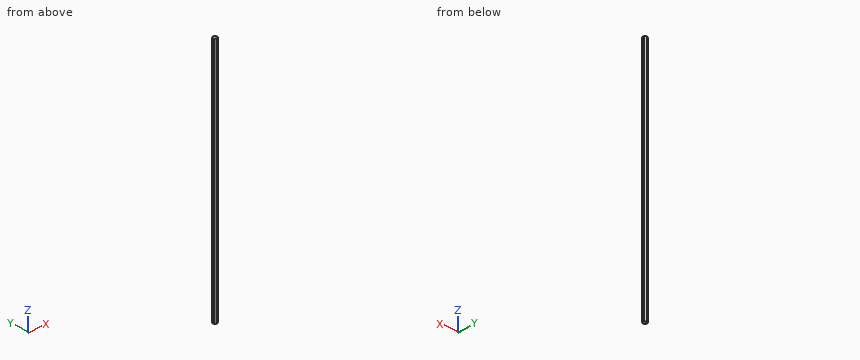
Autodesk Inventor part; units mm, degrees
ref_plane "YZ Plane" through (0, 0, 0) normal (1, 0, 0) x (0, 1, 0)
ref_plane "XZ Plane" through (0, 0, 0) normal (0, 1, 0) x (-1, 0, 0)
ref_plane "XY Plane" through (0, 0, 0) normal (0, 0, 1) x (1, 0, 0)
sketch "Sketch1" plane through (-2.1, -1.2124, 67.5) normal (0, 0, 1) x (1, 0, 0)
  line L0 (2.1, 4.0992) -> (4.6, 2.6558)
  line L1 (2.1, 3.6373) -> (0, 2.4249)
  line L2 (-0.4, 2.6558) -> (2.1, 4.0992)
  line L3 (-0.4, -0.2309) -> (-0.4, 2.6558)
  line L4 (2.1, -1.6743) -> (-0.4, -0.2309)
  line L5 (4.6, -0.2309) -> (2.1, -1.6743)
  line L6 (4.6, 2.6558) -> (4.6, -0.2309)
  point P0 (2.1, 1.2124)
extrude "Extrusion1" add sketch "Sketch1" against normal blind 317.5
sketch "Sketch2" plane through (-2.1, -1.2124, -250) normal (0, 0, -1) x (1, 0, 0)
  point P0 (2.1, -1.2124)
  point P1 (2.1, -1.2124)
properties part number "5mm axel"
Geometry: final body of the model. Coordinates: model frame, mm. Round coordinates to 2 decimals unless told otherwise and drop trailing zeros. Write each loop counter-clockwise with the first axis right and the second up, starting at its lowest first coordinate (ties: lowest second). Pieces come first, ordered by that corner, then holes. Notation, with made-up numbers: M 54.5,42.25 L 72.5,42.25 A31 cw 72.5,69.25 Z; hole C -32,-8.5 d3. An arc over 180 degrees is marked long. Write item = value, one per line.
Item 1: Material intervals for line 1 along Y through (x, z) = (-0.6, -142.5); line 2 along X through (y, z) = (1.8, -88.5); line 3 along X through (y, z) = (1.75, -161.5), sorted ascending. Write a range as [from, to].
Findings:
line_1 = [-2.54, 2.54]
line_2 = [-1.88, 1.88]
line_3 = [-1.97, 1.97]
Item 2: Section query A-A on z = 27.5. Return loops of the section in (x, y), then the cut area to 3 significant figures.
Findings:
outline = M -2.5,-1.44 L 0,-2.89 L 2.5,-1.44 L 2.5,1.44 L 0,2.89 L -2.5,1.44 Z
area = 21.7 mm^2
Item 3: Section query B-B on x = -1.7. Return loops of the section in (y, z), then the cut area to 3 significant figures.
Findings:
outline = M -1.91,-250 L 1.91,-250 L 1.91,67.5 L -1.91,67.5 Z
area = 1,210 mm^2
Item 4: Pin query (flat end, axial travel): P1, Ø1, axis at x = 1, z = -140, coming from the +Y side. Return the tip coordinate at first contact, or that it passes through.
Findings:
P1 = 2.6
